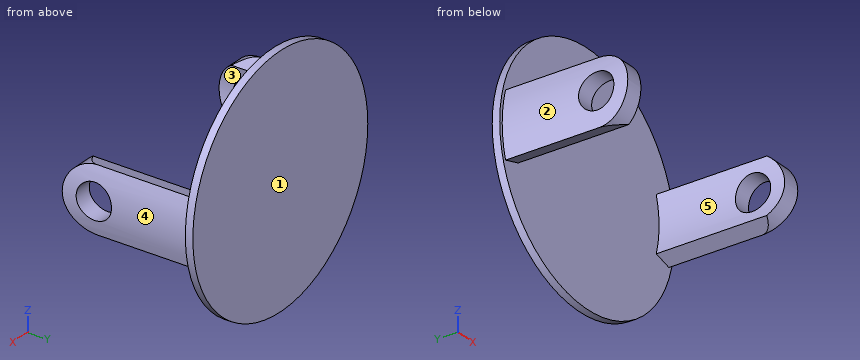
Autodesk Inventor part; units mm, degrees
ref_plane "to_trmnl_hold_XY" through (0, 0, 0) normal (0, -1, 0) x (1, 0, 0)
ref_plane "to_trmnl_hold_YZ" through (0, 0, 0) normal (1, 0, 0) x (0, 0, 1)
ref_plane "to_trmnl_hold_ZX" through (0, 0, 0) normal (0, 0, 1) x (0, -1, 0)
sketch "Sketch_2" plane through (0, 0, 0) normal (0, 1, 0) x (-1, 0, 0)
  circle A0 centre (0, 0) radius 4.064
extrude "Extrusion1" add sketch "Sketch_2" along normal blind 0.254
sketch "Sketch_3" plane through (0, 0, 0) normal (0, 1, 0) x (-1, 0, 0)
  arc A0 (-3.2099, 0.9236) -> (-3.2099, -0.9236) centre (0, 0) ccw
  line L0 (-3.2099, 0.9236) -> (-3.7957, 1.0922)
  arc A1 (-3.7957, 1.0922) -> (-3.7957, -1.0922) centre (0, 0) ccw
  line L1 (-3.7957, -1.0922) -> (-3.2099, -0.9236)
extrude "Extrusion2" add sketch "Sketch_3" against normal blind 4.2418
sketch "Sketch_4" plane through (0, 0, 0) normal (0, 1, 0) x (-1, 0, 0)
  arc A0 (3.7957, -1.0922) -> (3.7957, 1.0922) centre (0, 0) ccw
  line L0 (3.7957, 1.0922) -> (3.2099, 0.9236)
  arc A1 (3.2099, -0.9236) -> (3.2099, 0.9236) centre (0, 0) ccw
  line L1 (3.2099, -0.9236) -> (3.7957, -1.0922)
extrude "Extrusion3" add sketch "Sketch_4" against normal blind 4.2418
sketch "Sketch_5" plane through (0, 0, 0) normal (1, 0, 0) x (0, 1, 0)
  circle A0 centre (-3.175, 0) radius 0.5969
extrude "Extrusion4" cut sketch "Sketch_5" along normal mid plane 16.3576
sketch "Sketch_6" plane through (0, 0, 0) normal (1, 0, 0) x (0, 1, 0)
  line L0 (-4.4958, 1.0922) -> (-4.4958, -1.0922)
  line L1 (-4.4958, -1.0922) -> (-3.175, -1.0922)
  arc A0 (-3.175, 1.0922) -> (-3.175, -1.0922) centre (-3.1493, 0) ccw
  line L2 (-3.175, 1.0922) -> (-4.4958, 1.0922)
extrude "Extrusion5" cut sketch "Sketch_6" along normal mid plane 16.3576
ref_plane "to_trmnl_hold_XY" through (0, 0, 0) normal (0, -1, 0) x (1, 0, 0)
ref_plane "to_trmnl_hold_YZ" through (0, 0, 0) normal (1, 0, 0) x (0, 0, 1)
ref_plane "to_trmnl_hold_ZX" through (0, 0, 0) normal (0, 0, 1) x (0, -1, 0)
properties part number "SB4011NO-trmnls"
Check sheet for the modelled part. Datum: model origin and axes. Units: mm. Face numbers are marked on the shaded views. A direction names the side the tool comes from. Give positions to 0.01 mm unless a question says otherwise; leave off trailing zeros. Write each loop counter-clockwise with the first axis right and the second up, starting at its lowest first coordinate (ties: lowest second). Pieces come first, ordered by that corner, then holes. Notation, with made-up numbers: (-20.5, 36.5) -> (-15.5, 36.5) arc R28 ccw to (-15.5, 54.5) -> close; hole circle Ø3 at (80.5, 6.5). An arc over 180 degrees is marked (long way). One line per item, written item: value. Start each with the question number.
Item 1: Section check B-B on y = -2.9. Record the cut outline in (x, z), then the cut area to 3 significant figures.
Item 2: Tool access check on the marked faces 4 and 5. Record the directions out of +Z, -Z, +X, -X, +Y, -Y that give a thin tool (end or side, any length) a straight path to the whole face; none if there is none.
Item 3: Material ranges on probe 1 along Y at (x, z) = (-3.45, 0); probe 2 along Y at (x, z) = (-1, -0.75); probe 3 along X at (y, z) = (-2.05, -0.25), recorded low to high. Write a range as from..to.
Item 4: Section check A-A on y = -2. Record the cut outline in (x, z).
Item 5: Section check C-C on z = -0.25. Record the cut outline in (x, y).
Item 6: Section check D-D on x = 0. Record the cut outline in (y, z).
Item 7: Draft check along Z on the marked faces 1, 2 and 3. Enter one of: +Z half, -Z half, draft (parallel to the pull), parting line (faces both ways), or undercut.
Item 8: Gauge pin test, flat ends, axial feed: pin 1 (1.4 mm diameter, centred on y = -3.175, z = 0, fed in from +X); pin 2 (4 mm diameter, centred on x = -0.5, z = 1, fed in from -Y); pin 3 (1 mm diameter, centred on y = -3, z = 2, fed in from +X). Record the tip position at first contact, or that the pin passes through.
Results list:
1. outline: (-3.91, -0.53) arc R3.95 ccw to (-3.8, -1.09) -> (-3.21, -0.92) arc R3.34 cw to (-3.3, -0.53) -> close; (-3.91, 0.53) -> (-3.3, 0.53) arc R3.34 cw to (-3.21, 0.92) -> (-3.8, 1.09) arc R3.95 ccw to start; (3.21, -0.92) -> (3.8, -1.09) arc R3.95 ccw to (3.91, -0.53) -> (3.3, -0.53) arc R3.34 cw to start; (3.21, 0.92) arc R3.34 cw to (3.3, 0.53) -> (3.91, 0.53) arc R3.95 ccw to (3.8, 1.09) -> close
1. area: 1.19 mm²
2. face 4: +X, -Y
2. face 5: -Y
3. probe 1: -4.24..-3.77, -2.58..0.25
3. probe 2: 0..0.25
3. probe 3: -3.94..-3.33, 3.33..3.94
4. outline: (-3.8, -1.09) -> (-3.21, -0.92) arc R3.34 cw to (-3.21, 0.92) -> (-3.8, 1.09) arc R3.95 ccw to start; (3.21, -0.92) -> (3.8, -1.09) arc R3.95 ccw to (3.8, 1.09) -> (3.21, 0.92) arc R3.34 cw to start
5. outline: (-4.06, 0) -> (-3.94, 0) -> (-3.94, -2.63) -> (-3.33, -2.63) -> (-3.33, 0) -> (3.33, 0) -> (3.33, -2.63) -> (3.94, -2.63) -> (3.94, 0) -> (4.06, 0) -> (4.06, 0.25) -> (-4.06, 0.25) -> close; (-3.94, -4.21) -> (-3.33, -4.21) -> (-3.33, -3.72) -> (-3.94, -3.72) -> close; (3.33, -4.21) -> (3.94, -4.21) -> (3.94, -3.72) -> (3.33, -3.72) -> close
6. outline: (0, -4.06) -> (0.25, -4.06) -> (0.25, 4.06) -> (0, 4.06) -> close
7. face 1: draft
7. face 2: parting line
7. face 3: undercut
8. pin 1: x = 3.95
8. pin 2: y = 0
8. pin 3: through
